Geometry: final body of the model. Coordinates: model frame, mm. Face numbers are marked on the shaded views. A direction names the side the tool comes from. Give positions to 0.01 mm unless a question says otherwise; leave off trailing zeros. Write each loop counter-clockwise with the first axis right and the second up, starting at its lowest first coordinate (ties: lowest second). Pieces come first, ordered by that corner, then holes. Notation, with made-up numbers: (-8.75, 25) -> (26.25, 25) arc R24 ccw to (26.25, 41) -> close; hole circle Ø5 at (-31.5, 9). An arc over 180 degrees is marked (long way). Answer as a JSON object with one key per item and string values. Group by question number.
(1) Draft query along Z for the marked faces 1, 2 and 3. Return one class per face: +Z half, -Z half, draft (parallel to the pull), parting line (faces both ways), or undercut.
(2) Section query C-C on z = 0. State how many separate pieces and enclosed holes the cut face has, plus the area to 3 significant figures.
(3) Section query A-A on x = 0. Output: boundary loops of the cut face in (y, z).
(4) Section query B-B on z = -35. Output: boundary loops of the cut face in (x, y), plus the area to 3 significant figures.
(5) Contact query for flat-ended pins moving along their axis: pin 1 Ø4.5 at (x, y) = (-25, -3.5) entering from -Z; pin 2 Ø6 at (x, z) = (3, -6) entering from -Y; pin 3 Ø3 at (x, z) = (-10.5, -35.5) entering from -Y. Output: stop coordinate, or through.
(6) Set-up query: the marked faces 4, 5 and 6. Return all of +Z, -Z, +X, -X, +Y, -Y with unobstructed straight access to the full face (end or side cutting, diameter ignored); none if empty.
(7) Material intervals for probe 1 along Z at (x, y) = (1.5, 3.5); probe 2 along Y at (x, z) = (8, -11.5); probe 3 along Y at (x, z) = (-9.5, -16.5), sorted ascending.
from build123d import *
from OCP.BRepFilletAPI import BRepFilletAPI_MakeChamfer

# Parameters (mm, degrees)
SKETCH_1_R          = 55
EXTRUDE_1_DEPTH     = 5
SKETCH_2_R          = 49.9
EXTRUDE_2_DEPTH     = 5
SKETCH_3_W          = 35
SKETCH_3_H          = 30
EXTRUDE_3_DEPTH     = 25
SKETCH_4_W          = 20.2
SKETCH_4_H          = 10.3
CUT_EXTRUDE_1_DEPTH = 93.466210045
SKETCH_5_R          = 4.1
CUT_EXTRUDE_2_DEPTH = 82.700673192
CHAMFER1_SIZE       = 2
CHAMFER1_SIZE2      = 0.535898385
SKETCH2_W           = 35
SKETCH2_H           = 30
CUT_EXTRUDE1_DEPTH  = 12.5
BOSS_EXTRUDE1_START = -2
SKETCH4_W           = 70
SKETCH4_H           = 20
BOSS_EXTRUDE1_DEPTH = 5.35
SKETCH5_R           = 4.15
CUT_EXTRUDE2_DEPTH  = 80.281917882
CUT_EXTRUDE3_DEPTH  = 6.5
CHAMFER2_SIZE       = 1
CHAMFER2_SIZE2      = 2.747477419


with BuildPart() as part:
    # Эскиз1 → Бобышка-Вытянуть1 (new body)
    with BuildSketch(Plane(origin=(0, 0, 0), x_dir=(1, 0, 0), z_dir=(0, 1, 0))):
        with Locations(Location((0, 0, 0), (0, 0, 270))):
            Circle(SKETCH_1_R)
    extrude(amount=EXTRUDE_1_DEPTH)

    # Эскиз2 → Бобышка-Вытянуть2 (add)
    with BuildSketch(Plane(origin=(0, 5, 0), x_dir=(1, 0, 0), z_dir=(0, 1, 0))):
        with Locations(Location((0, 0, 0), (0, 0, 270))):
            Circle(SKETCH_2_R)
    extrude(amount=EXTRUDE_2_DEPTH)

    # Эскиз3 → Бобышка-Вытянуть3 (add)
    with BuildSketch(Plane.XZ):
        Rectangle(SKETCH_3_W, SKETCH_3_H)
    extrude(amount=EXTRUDE_3_DEPTH)

    # Эскиз4 → Вырез-Вытянуть1 (cut, through all)
    with BuildSketch(Plane.XY.offset(15)):
        with Locations((0, -12.5)):
            Rectangle(SKETCH_4_W, SKETCH_4_H)
    extrude(amount=-CUT_EXTRUDE_1_DEPTH, mode=Mode.SUBTRACT)

    # Эскиз5 → Вырез-Вытянуть2 (cut, through all)
    with BuildSketch(Plane.XZ):
        with Locations(Location((33.592198598, -32.871936263, 0), (0, 0, 270))):
            Circle(SKETCH_5_R)
        with Locations(Location((-33.591727056, -32.872418125, 0), (0, 0, 270))):
            Circle(SKETCH_5_R)
        with Locations(Location((-33.591727056, 32.872418125, 0), (0, 0, 270))):
            Circle(SKETCH_5_R)
        with Locations(Location((33.483215177, 32.983215177, 0), (0, 0, 270))):
            Circle(SKETCH_5_R)
    extrude(amount=-CUT_EXTRUDE_2_DEPTH, mode=Mode.SUBTRACT)

    # Chamfer1: one chamfer whose edges measure the first distance from different faces: ONE call of the kernel's chamfer builder (chamfer() names one face for all edges)
    chamfer1_edges_1 = [part.edges().sort_by_distance(p)[0] for p in [
        (0.000357897, 10, -49.899999999),
    ]]
    chamfer1_side_1 = [part.faces().sort_by_distance(p)[0] for p in [
        (0.000357897, 7.5, -49.899999999),
    ]]
    chamfer1_edges_2 = [part.edges().sort_by_distance(p)[0] for p in [
        (-49.9, 10, 0),
    ]]
    chamfer1_side_2 = [part.faces().sort_by_distance(p)[0] for p in [
        (-49.9, 7.5, 0),
    ]]
    chamfer1_edges_3 = [part.edges().sort_by_distance(p)[0] for p in [
        (-0.08242255, 10, 49.899931929),
    ]]
    chamfer1_side_3 = [part.faces().sort_by_distance(p)[0] for p in [
        (-0.08242255, 7.5, 49.899931929),
    ]]
    chamfer1_edges_4 = [part.edges().sort_by_distance(p)[0] for p in [
        (49.899931657, 10, 0.082587101),
    ]]
    chamfer1_side_4 = [part.faces().sort_by_distance(p)[0] for p in [
        (49.899931657, 7.5, 0.082587101),
    ]]
    chamfer1 = BRepFilletAPI_MakeChamfer(part.part.solid().wrapped)
    for e in chamfer1_edges_1:
        chamfer1.Add(CHAMFER1_SIZE, CHAMFER1_SIZE2, e.wrapped, chamfer1_side_1[0].wrapped)  # the first distance lies on this face
    for e in chamfer1_edges_2:
        chamfer1.Add(CHAMFER1_SIZE, CHAMFER1_SIZE2, e.wrapped, chamfer1_side_2[0].wrapped)  # the first distance lies on this face
    for e in chamfer1_edges_3:
        chamfer1.Add(CHAMFER1_SIZE, CHAMFER1_SIZE2, e.wrapped, chamfer1_side_3[0].wrapped)  # the first distance lies on this face
    for e in chamfer1_edges_4:
        chamfer1.Add(CHAMFER1_SIZE, CHAMFER1_SIZE2, e.wrapped, chamfer1_side_4[0].wrapped)  # the first distance lies on this face
    add(Compound.cast(chamfer1.Shape()), mode=Mode.REPLACE)

    # Sketch2 → Cut-Extrude1 (cut)
    with BuildSketch(Plane.XZ.offset(25)):
        Rectangle(SKETCH2_W, SKETCH2_H)
    extrude(amount=-CUT_EXTRUDE1_DEPTH, mode=Mode.SUBTRACT)

    # Sketch4 → Boss-Extrude1 (add)
    with BuildSketch(Plane.XZ.offset(7.35).offset(BOSS_EXTRUDE1_START)):
        Rectangle(SKETCH4_W, SKETCH4_H)
    extrude(amount=-BOSS_EXTRUDE1_DEPTH)

    # Sketch5 → Cut-Extrude2 (cut, through all)
    with BuildSketch(Plane.XZ.offset(5.35)):
        with Locations((25, 0)):
            Circle(SKETCH5_R)
        with Locations((-25, 0)):
            Circle(SKETCH5_R)
    extrude(amount=-CUT_EXTRUDE2_DEPTH, mode=Mode.SUBTRACT)

    # Sketch6 → Cut-Extrude3 (cut)
    with BuildSketch(Plane(origin=(0, 10, 0), x_dir=(1, 0, 0), z_dir=(0, 1, 0))):
        Polygon((-18.504809472, 3.75), (-25, 7.5), (-31.495190528, 3.75), (-31.495190528, -3.75), (-25, -7.5), (-18.504809472, -3.75), align=None)
        Polygon((31.495190528, 3.75), (25, 7.5), (18.504809472, 3.75), (18.504809472, -3.75), (25, -7.5), (31.495190528, -3.75), align=None)
    extrude(amount=-CUT_EXTRUDE3_DEPTH, mode=Mode.SUBTRACT)

    # Chamfer2
    chamfer2_edges = [part.edges().sort_by_distance(p)[0] for p in [
        (-18.504809472, 10, 0),
        (-21.752404736, 10, -5.625),
        (-28.247595264, 10, -5.625),
        (-31.495190528, 10, 0),
        (-28.247595264, 10, 5.625),
        (-21.752404736, 10, 5.625),
        (31.495190528, 10, 0),
        (28.247595264, 10, -5.625),
        (21.752404736, 10, -5.625),
        (18.504809472, 10, 0),
        (21.752404736, 10, 5.625),
        (28.247595264, 10, 5.625),
    ]]
    chamfer2_side = [part.faces().sort_by_distance(p)[0] for p in [
        (0.000665728, 10, -0.000672626),
    ]]
    chamfer(chamfer2_edges, length=CHAMFER2_SIZE, length2=CHAMFER2_SIZE2, reference=chamfer2_side[0])


solid = part.part
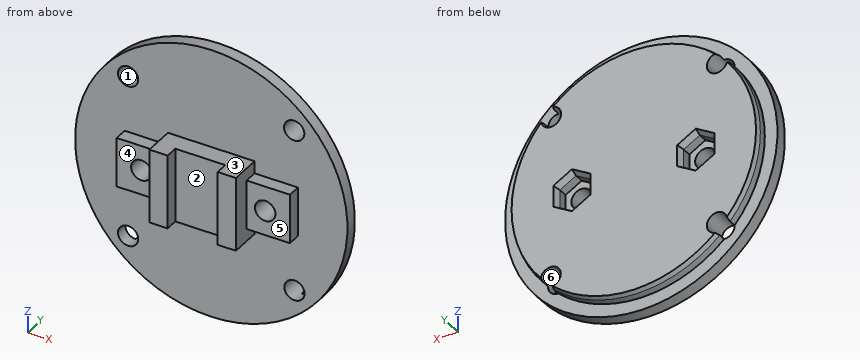
Answer list:
{
 "1": {"face 1": "undercut", "face 2": "draft", "face 3": "+Z half"},
 "2": {"separate pieces": "3", "enclosed holes": "0", "area": "1,250 mm2"},
 "3": {"outline": "(-7.35, -15) -> (0, -15) -> (0, -55) -> (5, -55) -> (5, -49.9) -> (8, -49.9) -> (10, -49.36) -> (10, 49.36) -> (8, 49.9) -> (5, 49.9) -> (5, 55) -> (0, 55) -> (0, 15) -> (-7.35, 15) -> close"},
 "4": {"outline": "(-42.43, 0) -> (-37.1, 0) -> (-37.1, 5) -> (-42.43, 5) -> close; (-30.09, 0) -> (30.09, 0) -> (30.09, 10) -> (-30.09, 10) -> close; (37.1, 0) -> (42.43, 0) -> (42.43, 5) -> (37.1, 5) -> close", "area": "655 mm2"},
 "5": {"pin 1": "z = -10", "pin 2": "y = -7.35", "pin 3": "y = 0"},
 "6": {"face 4": "+Z, -Z, -X, -Y", "face 5": "+Z, -Z, +X, -Y", "face 6": "+Y, -Y"},
 "7": {"probe 1": "-54.98 to 54.98", "probe 2": "-7.35 to 10", "probe 3": "0 to 10"}
}
